Read the model definition and answer for the solid it produces. Units are mm, in the model's axes. Coordinates: 2 decimals unless noted, no trailing zeros. Order: outer loops, then holes, each group sorted by start corner. A loop starts at its lowest first (then second) coordinate and runs counter-clockwise, first axis right, second up. Notation, with made-up numbers: (26, 52) -> (55, 52) arc R21 cw to (55, 62) -> close; hole circle Ø3 at (71.5, 9). An arc over 180 degrees is marked (long way). Answer as a JSON object with one key per item and string values. Group by question number.
1) Section A-A on z = 8 is taken. Determine the outline of the cut face in (x, y), and give its area (3 significant figures).
2) Determine the mould class of faces 1 (the flat face through (1, -1, 22.2)), 2 (the cylindrical face through (0, 2, 11)), 3 (the conical face through (0, 0, 1)) for opening direction Y: released by +Y, released by -Y, zero draft, split by the parting line, or undercut.
3) Consider L1, parallel to X at y = -0.1, z = 20.5; L2, parallel to Y at x = 0.5, z = 17; L3, parallel to X at y = -1.65, z = 20.75. Determine where each line is inside the solid, lowest interval first.
Autodesk Inventor part; units mm, degrees
ref_plane "YZ Plane" through (0, 0, 0) normal (1, 0, 0) x (0, 1, 0)
ref_plane "XZ Plane" through (0, 0, 0) normal (0, 1, 0) x (-1, 0, 0)
ref_plane "XY Plane" through (0, 0, 0) normal (0, 0, 1) x (1, 0, 0)
sketch "Sketch1" plane through (0, 0, 0) normal (0, 0, 1) x (1, 0, 0)
  circle A0 centre (0, 0) radius 2
  dimension "d0" = 4
extrude "Extrusion1" add sketch "Sketch1" along normal blind 22.2
chamfer "Chamfer1" distance 0.25 angle 45 2 edges at (-2, 0, 22.2) (-2, 0, 0)
sketch "Sketch2" plane through (0, 0, 0) normal (1, 0, 0) x (0, 1, 0)
  line L0 (2, 0.25) -> (1.75, 0)
  line L1 (1.75, 0) -> (-1.75, 0)
  line L2 (-1.75, 0) -> (-2, 0.25)
  line L3 (-2, 0.25) -> (-2, 21.95)
  line L4 (-2, 21.95) -> (-1.75, 22.2)
  line L5 (-1.75, 22.2) -> (1.75, 22.2)
  line L6 (1.75, 22.2) -> (2, 21.95)
  line L7 (2, 21.95) -> (2, 0.25)
  line L8 (-1.75, 22.2) -> (1.75, 22.2)
  line L9 (1, 22.2) -> (0, 21.2)
  line L10 (0, 21.2) -> (0, 22.2)
  line L11 (1, 0) -> (0, 1)
  line L12 (0, 1) -> (0, 0)
  line L13 (0, -4.4) -> (0, 26.4)
  dimension "d6" = 1
  dimension "d7" = 1
  dimension "d8" = 45
revolve "Revolution1" cut sketch "Sketch2" angle 360 about axis through (0, 0, -10) along (0, 0, 1) contours L1 L12 L11 | L9 L10 L5
properties part number "MotorBeltTensionerAxis"
Worked answers:
{
 "1": {"outline": "circle Ø4 at (0, 0)", "area": "12.6 mm²"},
 "2": {"face 1": "zero draft", "face 2": "split by the parting line", "face 3": "undercut"},
 "3": {"L1": "x = -2 to 2", "L2": "y = -1.94 to 1.94", "L3": "x = -1.13 to 1.13"}
}
